Can you work these out from the drawing? Everything is in mm from the part's minimum corner. A direction names the side the tool comes from. Round coordinates to 2 decimals unless told otherwise and drop trailing zeros. Write each loop counter-clockwise with the first axis right and the second up, starting at its lowest first coordinate (ties: lowest second). Pieces come first, ordered by that corner, then holes. Notation, with made-up numbers: M -11.5,76 L 33.5,76 A29 cw 33.5,115 Z; hole C 85.5,8.25 d10. An arc over 180 degrees is marked long. Answer in a Markdown table with one row per item. Add a question column.
(1) Suppose I cut it at A-A, the plane x = 13.5. Write out the boundary of the cut face in (y, z) (1 decimal).
(2) I'm going to push a flat-ended pin straight in: pin 1 (1.4 mm diameter, centred on x = 12.95, y = 2.89, fed in from -Z). Where does the tip first touch, or does it pass through?
(3) For the marked faces 4 and 5, which set-ups out of +Z, -Z, +X, -X, +Y, -Y let a thin tool reach every point of the face, with its end or its side?
(4) Suppose I cut it at D-D, the plane z = 0.75. Count the separate pieces of the cut face and the enclosed holes in it.
(5) If we mould it in two halves opening along X, with no side actions, what happens to the marked faces 1, 2 and 3? For each: released by +X, released by -X, zero draft, split by the parting line, or undercut.
(6) If I drill on probe 1 along Y at (x, z) = (12.95, 0.7) (1 decimal); probe 2 along Y at (x, z) = (13.5, 0.2) (1 decimal); probe 3 along X at (y, z) = (9.25, 0.2), over which ranges is the centre line in solid material (lowest first)?
(7) Suppose I cut it at B-B, the plane y = 10.75. Write out the boundary of the cut face in (x, z).
(8) Suppose I cut it at C-C, the plane x = 16. Write out the boundary of the cut face in (y, z).
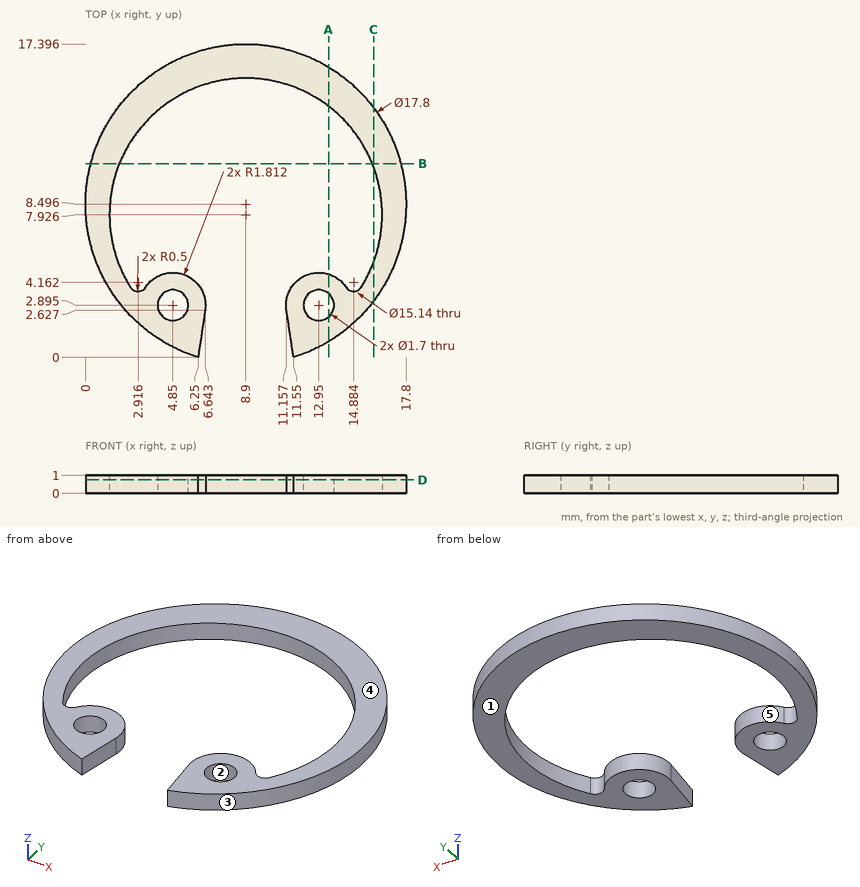
Calculated:
| question | item | result |
|---|---|---|
| 1 | outline | M 0.9,0 L 2.2,0 L 2.2,1 L 0.9,1 Z; M 3.5,0 L 4.6,0 L 4.6,1 L 3.5,1 Z; M 13.9,0 L 16.1,0 L 16.1,1 L 13.9,1 Z |
| 2 | pin 1 | through |
| 3 | face 4 | +Z, +X, -X, +Y, -Y |
| 3 | face 5 | +Z, -Z |
| 4 | separate pieces | 1 |
| 4 | enclosed holes | 2 |
| 5 | face 1 | zero draft |
| 5 | face 2 | undercut |
| 5 | face 3 | split by the parting line |
| 6 | probe 1 | 0.6 to 2, 3.7 to 4.7, 14.3 to 16.4 |
| 6 | probe 2 | 0.9 to 2.2, 3.5 to 4.6, 13.9 to 16.1 |
| 6 | probe 3 | 0.03 to 1.45, 16.35 to 17.77 |
| 7 | outline | M 0.29,0 L 1.88,0 L 1.88,1 L 0.29,1 Z; M 15.92,0 L 17.51,0 L 17.51,1 L 15.92,1 Z |
| 8 | outline | M 3.13,0 L 5.3,0 L 5.3,1 L 3.13,1 Z; M 10.55,0 L 13.86,0 L 13.86,1 L 10.55,1 Z |
